from build123d import *

# Parameters (mm, degrees)
F0_R     = 12.8905
F0_R_2   = 11.43
F0_R_3   = 6.5405
F1_DEPTH = 19.05
F2_R     = 34.92499


# Not quite as in the source:
# - a fillet or chamfer is up to 0.001 mm smaller than in the source, because OpenCascade refuses the exact size


with BuildPart() as f1:
    # F0 (on Top) → F1 (new body)
    with BuildSketch(Plane.XY):
        with BuildLine():
            Line((421.005, 38.1), (0, 38.1))
            ThreePointArc((0, 38.1), (-34.925, 3.175), (0, -31.75))
            Line((0, -31.75), (421.005, -31.75))
            Line((421.005, -31.75), (421.005, 38.1))
        make_face()
        Circle(F0_R, mode=Mode.SUBTRACT)
        with Locations((48.26, 15.875)):
            Circle(F0_R_2, mode=Mode.SUBTRACT)
        with Locations((74.168, 15.875)):
            Circle(F0_R_2, mode=Mode.SUBTRACT)
        with Locations((99.822, 15.875)):
            Circle(F0_R_2, mode=Mode.SUBTRACT)
        with Locations((125.476, 15.875)):
            Circle(F0_R_2, mode=Mode.SUBTRACT)
        with Locations((324.485, 3.175)):
            Circle(F0_R_3, mode=Mode.SUBTRACT)
        with Locations((387.985, 3.175)):
            Circle(F0_R_3, mode=Mode.SUBTRACT)
    extrude(amount=F1_DEPTH)

    # F2 (radius 34.925 in the source; OpenCascade refuses exactly that, so slightly less here)
    f2_edges = [f1.edges().sort_by_distance(p)[0] for p in [
        (421.005, 38.1, 9.525),
        (421.005, -31.75, 9.525),
    ]]
    fillet(f2_edges, radius=F2_R)


solid = f1.part
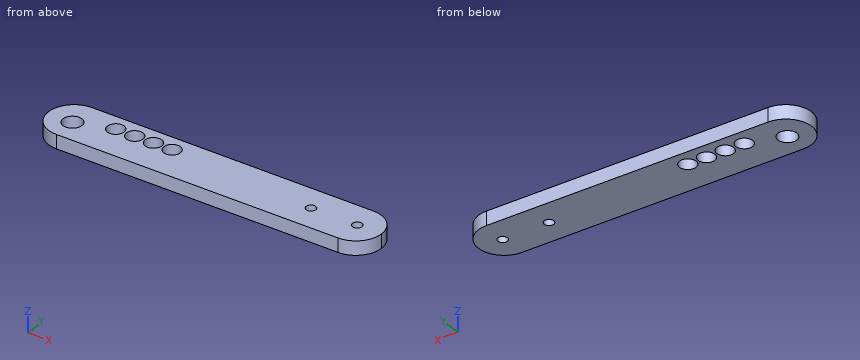
For this review, take the finished solid that the model builds, in its own axes (mm). Coordinates: 2 decimals unless noted, no trailing zeros. Order: outer loops, then holes, each group sorted by start corner. A loop starts at its lowest first (then second) coordinate and runs counter-clockwise, first axis right, second up. Notation, with made-up numbers: (22.25, 22.25) - (48.25, 22.25) arc R28 cw to (48.25, 57.25) - close; hole circle Ø2 at (-40, 20). An arc over 180 degrees is marked (long way). Answer as CSV lines item,"result". Start each with the question number.
1) Add section B-B (y = -9). State the section outline as (x, z) points.
2) Add section C-C (z = 11.75). Count the separate pieces of the cut face and the enclosed holes in it, then the cut area to 3 significant figures.
3) Insertion check: P1, Ø17, axis at x = 324.485, y = 3.175, coming from the +Z side; P2, Ø12, axis at x = 387.985, y = 3.175, coming from the +Z side; P3, Ø4, axis at y = -17, z = 10.5, coming from the +X side; P4, Ø10, axis at y = 28, z = 16, coming from the +X side. Each pin has a flat end and moves straight along its axis. Give the tip position at first contact, or say it passes through.
4) To check wall thickness, follow line 1 along Y through (x, z) = (48.26, 5) (3 decimals); line 2 along X through (y, z) = (18, 4.25); line 3 along X through (y, z) = (3.5, 2). State the ranges of each line that lie inside material, in increasing order. Write a range as [from, to].
5) Add section A-A (x = 48.26). State the section outline as (y, z) points (3 decimals), then the cut area to 3 significant figures.
6) Add section D-D (y = 23). State the section outline as (x, z) points, then the cut area to 3 significant figures.
Result:
1,outline,"(-32.73, 0) - (-9.23, 0) - (-9.23, 19.05) - (-32.73, 19.05) - close; (9.23, 0) - (418.81, 0) - (418.81, 19.05) - (9.23, 19.05) - close"
2,separate pieces,"1"
2,enclosed holes,"7"
2,area,"28,400 mm^2"
3,P1,"z = 19.05"
3,P2,"through"
3,P3,"x = 415.9"
3,P4,"x = 414.83"
4,line 1,"[-31.75, 4.445], [27.305, 38.1]"
4,line 2,"[-31.62, 37.03], [59.49, 62.94], [85.4, 88.59], [111.05, 114.25], [136.71, 417.7]"
4,line 3,"[-34.92, -12.41], [12.41, 317.95], [331.02, 381.45], [394.52, 421]"
5,outline,"(-31.75, 0) - (4.445, 0) - (4.445, 19.05) - (-31.75, 19.05) - close; (27.305, 0) - (38.1, 0) - (38.1, 19.05) - (27.305, 19.05) - close"
5,area,"895 mm^2"
6,outline,"(-28.75, 0) - (39.32, 0) - (39.32, 19.05) - (-28.75, 19.05) - close; (57.2, 0) - (65.23, 0) - (65.23, 19.05) - (57.2, 19.05) - close; (83.11, 0) - (90.88, 0) - (90.88, 19.05) - (83.11, 19.05) - close; (108.76, 0) - (116.54, 0) - (116.54, 19.05) - (108.76, 19.05) - close; (134.41, 0) - (414.83, 0) - (414.83, 19.05) - (134.41, 19.05) - close"
6,area,"7,090 mm^2"
